Input: part model. Units: mm. Frame: model coordinates. Face numbers are marked on the shaded views. A direction names the side the tool comes from. Round coordinates to 2 decimals unless told otherwise and drop trailing zeros. Loops run counter-clockwise (first coordinate to the right, second up) from the corner with the lowest first, then second, coordinate; pieces in that order, holes last. Notation, with made-up numbers: M 8,49 L 24,49 A16 cw 24,65 Z; hole C 56.5,81 d7. An arc over 180 degrees is marked long. Use one line per item in the form item = value. Start each with the question number.
Q1. Section query A-A, the plane x = 15. Output: boundary loops of the cut face in (y, z), and give its area (3 significant figures).
Q2. Section query D-D, the plane x = 0. Output: boundary loops of the cut face in (y, z).
Q3. Ray query, line 1 along Z through (x, y) = (-15, 1.65); line 2 along Z through (x, y) = (-3.5, 6.5); line 3 along Y through (x, z) = (13.5, 2). Return the intervals inside material, ascending.
Q4. Section query C-C, the plane y = 2. Output: boundary loops of the cut face in (x, z).
Q5. Access query for the marked faces 1, 2, 3, 4 and 5. Directions: +Z, -Z, +X, -X, +Y, -Y. A direction counts if a zero-diameter tool reaches every point of the face in a straight line with its end or side. Return the directions, or none.
Q6. Section query B-B, the plane z = 13.5. Output: boundary loops of the cut face in (x, y), and give its area (3 significant figures).
Q7. First-contact query: P1, Ø2, axis at x = -2, y = 2.5, coming from the +Z side (3 decimals); P2, Ø5, axis at y = 9, z = 6, coming from the -X side; P3, Ø2, axis at x = 15.5, z = 11, coming from the +Y side; P4, Ø1, axis at y = 8, z = 17, coming from the -X side. Flat tips, straight axial feed; report the tip coordinate or a pass-through.
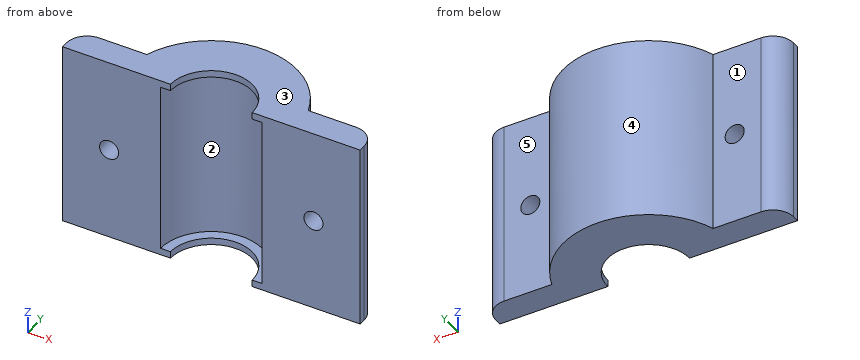
```python
from build123d import *

# Parameters (mm, degrees)
SKETCH006_R  = 1.4
PAD004_DEPTH = 4
PAD_DEPTH    = 27
PAD001_DEPTH = 1
PAD003_DEPTH = 1
FILLET_R     = 3


with BuildPart() as mount:
    # Sketch006 → Pad004 (new body)
    with BuildSketch(Plane.XZ):
        with Locations((-15, 13.5)):
            Circle(SKETCH006_R)
        with Locations((15, 13.5)):
            Circle(SKETCH006_R)
    extrude(amount=-PAD004_DEPTH)


with BuildPart() as base:
    # Sketch → Pad (new body)
    with BuildSketch(Plane.XY):
        with BuildLine():
            ThreePointArc((7.45, 0), (0, 7.45), (-7.45, 0))
            Line((-7.45, 0), (-21.842719, 0))
            Line((-21.842719, 0), (-21.842719, 4))
            Line((-21.842719, 4), (-11.842719, 4))
            ThreePointArc((11.842719, 4), (0, 12.5), (-11.842719, 4))
            Line((21.842719, 4), (11.842719, 4))
            Line((21.842719, 0), (21.842719, 4))
            Line((7.45, 0), (21.842719, 0))
        make_face()
    extrude(amount=PAD_DEPTH)


with BuildPart() as bottomlip:
    # Sketch003 → Pad001 (new body)
    with BuildSketch(Plane.XY):
        with BuildLine():
            ThreePointArc((7.46, 0), (0, 7.46), (-7.46, 0))
            Line((-7.46, 0), (-6, 0))
            ThreePointArc((6, 0), (0, 6), (-6, 0))
            Line((7.46, 0), (6, 0))
        make_face()
    extrude(amount=PAD001_DEPTH)


with BuildPart() as fillet_body:
    # Sketch005 → Pad003 (new body)
    with BuildSketch(Plane.XY.offset(26)):
        with BuildLine():
            ThreePointArc((7.46, 0), (0, 7.46), (-7.46, 0))
            Line((-7.46, 0), (-6, 0))
            ThreePointArc((6, 0), (0, 6), (-6, 0))
            Line((7.46, 0), (6, 0))
        make_face()
    extrude(amount=PAD003_DEPTH)

    # Fusion: union Base, BottomLip
    add(base.part)
    add(bottomlip.part)

    # Cut: cut Mount
    add(mount.part, mode=Mode.SUBTRACT)

    # Fillet
    fillet_edges = [fillet_body.edges().sort_by_distance(p)[0] for p in [
        (21.842719, 4, 13.5),
        (-21.842719, 4, 13.5),
    ]]
    fillet(fillet_edges, radius=FILLET_R)


solid = fillet_body.part
```
Results found:
q1.outline = M 0,0 L 4,0 L 4,12.1 L 0,12.1 Z; M 0,14.9 L 4,14.9 L 4,27 L 0,27 Z
q1.area = 96.8 mm²
q2.outline = M 6,0 L 12.5,0 L 12.5,27 L 6,27 L 6,26 L 7.45,26 L 7.45,1 L 6,1 Z
q3.line_1 = 0 to 12.1, 14.9 to 27
q3.line_2 = 0 to 1, 26 to 27
q3.line_3 = 0 to 4
q4.outline = M -21.67,0 L -5.66,0 L -5.66,1 L -7.18,1 L -7.18,26 L -5.66,26 L -5.66,27 L -21.67,27 Z; M 5.66,0 L 21.67,0 L 21.67,27 L 5.66,27 L 5.66,26 L 7.18,26 L 7.18,1 L 5.66,1 Z; hole C -15,13.5 d2.8; hole C 15,13.5 d2.8
q5.face_1 = +Z, -Z, -X, +Y
q5.face_2 = -Y
q5.face_3 = +Z, +X, -X, +Y, -Y
q5.face_4 = +Z, -Z, +Y
q5.face_5 = +Z, -Z, +X, +Y
q6.outline = M -21.84,0 L -16.4,0 L -16.4,4 L -18.84,4 A3 ccw -21.84,1 Z; M -13.6,0 L -7.45,0 A7.45 cw 7.45,0 L 13.6,0 L 13.6,4 L 11.84,4 A12.5 ccw -11.84,4 L -13.6,4 Z; M 16.4,0 L 21.84,0 L 21.84,1 A3 ccw 18.84,4 L 16.4,4 Z
q6.area = 208 mm²
q7.P1 = through
q7.P2 = -10.68
q7.P3 = 4
q7.P4 = -10
